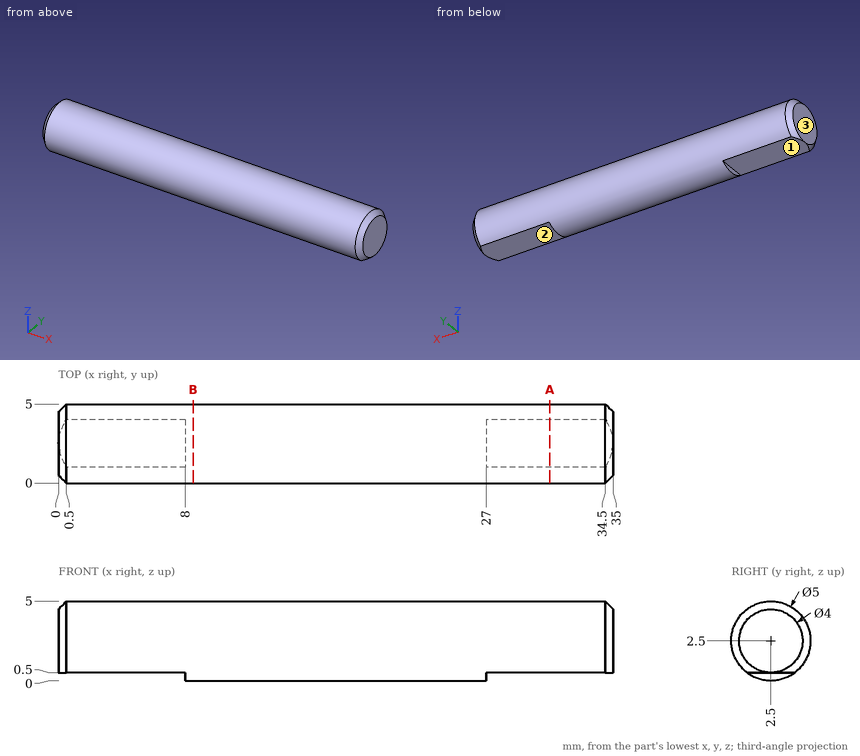
The drawing under review shows one solid part. Ordinate dimensions are in mm from its lowest x, y, z. A direction names the side the tool comes from. Give positions to 0.01 mm unless a question says otherwise; leave off trailing zeros. Loops run counter-clockwise (first coordinate to the right, second up) from the corner with the lowest first, then second, coordinate; pieces in that order, holes last. Notation, with made-up numbers: M -34.75,-20 L -3.75,-20 A29 cw -3.75,2 Z; hole C 67.5,51.25 d9. An arc over 180 degrees is marked long. One line per item, written item: value. Start each with the question number.
Q1. Add section B-B (x = 8.5). Give the boundary of the cut face in (y, z), and give its area (3 significant figures).
Q2. Clearance check with flat-ended pins moving along their axes: pin 1 Ø1.5 at (x, y) = (32.5, 2) entering from -Z; pin 2 Ø1 at (x, y) = (19, 3) entering from +Z. State where each tip first meets the part, or that it passes through.
Q3. For L1, parallel to Y at x = 31, z = 2.4; L2, parallel to Y at x = 18, z = 4.5, list the stretches that pass through material, from the lowest coordinate up.
Q4. Add section A-A (x = 31). Give the boundary of the cut face in (y, z).
Q5. Machinability: for the marked faces 1, 2 and 3, which of the approach directions +Z, -Z, +X, -X, +Y, -Y give a long, thin tool a straight path to every point of the face, cutting with its end or side? Answer none if there is none.
Reply:
1. outline: C 2.5,2.5 d5
1. area: 19.6 mm²
2. pin 1: z = 0.5
2. pin 2: z = 5
3. L1: 0 to 5
3. L2: 1 to 4
4. outline: M 1,0.5 L 4,0.5 A2.5 ccw long Z
5. face 1: -Z, -X, +Y, -Y
5. face 2: -Z, +X, +Y, -Y
5. face 3: +Z, -Z, -X, +Y, -Y
